Model file for the job. Use its own axes, mm. Face numbers are marked on the shaded views. Coordinates: 2 decimals unless noted, no trailing zeros. Write each loop counter-clockwise with the first axis right and the second up, starting at its lowest first coordinate (ties: lowest second). Pieces come first, ordered by that corner, then holes.
Q1. Pull direction Y, two halves, no side cores. Call the marked faces 1, 2, 3 and 4: released by +Y, released by -Y, zero draft, split by the parting line, or undercut.
Q2. Drill centre lines: probe 1 along Y at (x, z) = (755.5, 739); probe 2 along Y at (x, z) = (742, 731); probe 3 along X at (y, z) = (-300, 716.5). Where is each one in solid material? Low to high.
Q3. Band-saw the part on A-A, the plane y = -300. Write the cut outline in (x, z).
Q4. Band-saw the part on D-D, the plane x = 737. Write the cut outline in (y, z), plus the area to 3 significant figures.
Q5. Band-saw the part on C-C, the plane z = 742. Write the cut outline in (x, y).
Q6. Pin check, flat tips, straight feed: P1, Ø20, axis at y = -581, z = 729, coming from the -X side; P2, Ø4, axis at x = 744.5, z = 724, coming from the +Y side; P3, Ø6, axis at x = 750, y = -300, coming from the -Z side; P4, Ø12, axis at x = 744.5, y = -298, coming from the +Z side. Stop position of each tip, or through.
Q7. Band-saw the part on B-B, the plane z = 717. Write the cut outline in (x, y), plus the area to 3 significant figures.
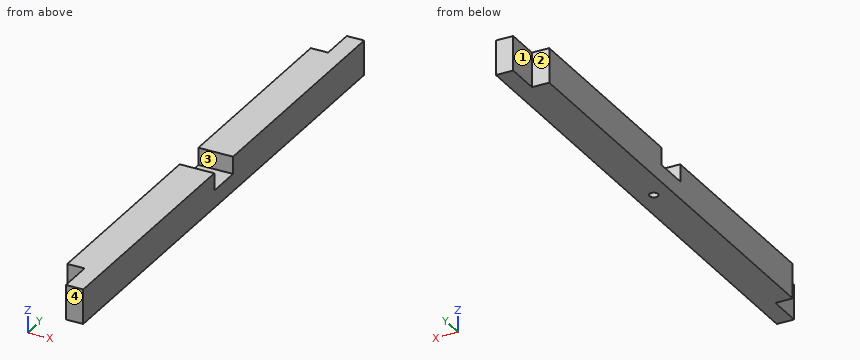
from build123d import *

# Parameters (mm, degrees)
SKETCH018_W     = 40
SKETCH018_H     = 40
PAD018_DEPTH    = 600
SKETCH019_W     = 40
SKETCH019_H     = 40
POCKET_DEPTH    = 20
SKETCH020_W     = 40
SKETCH020_H     = 40
POCKET001_DEPTH = 20
SKETCH064_R     = 5
POCKET019_DEPTH = 40.001


with BuildPart() as part:
    # Sketch018 → Pad018 (new body)
    with BuildSketch(Plane.XZ):
        with Locations((20, 280)):
            Rectangle(SKETCH018_W, SKETCH018_H)
    extrude(amount=PAD018_DEPTH)

    # Sketch019 (on Face4 of Pad018) → Pocket (cut)
    with BuildSketch(Plane(origin=(0, 0, 0), x_dir=(0, 0, -1), z_dir=(-1, 0, 0))):
        with Locations((-280, 580)):
            Rectangle(SKETCH019_W, SKETCH019_H)
        with Locations((-280, 20)):
            Rectangle(SKETCH019_W, SKETCH019_H)
    extrude(amount=-POCKET_DEPTH, mode=Mode.SUBTRACT)

    # Sketch020 (on Face1 of Pocket) → Pocket001 (cut)
    with BuildSketch(Plane(origin=(0, 0, 300), x_dir=(-1, 0, 0), z_dir=(0, 0, 1))):
        with Locations((-20, 300)):
            Rectangle(SKETCH020_W, SKETCH020_H)
    extrude(amount=-POCKET001_DEPTH, mode=Mode.SUBTRACT)

    # Sketch064 (on Face8 of Pocket001) → Pocket019 (cut, through all)
    with BuildSketch(Plane(origin=(0, 0, 260), x_dir=(1, 0, 0), z_dir=(0, 0, -1))):
        with Locations((20, 300)):
            Circle(SKETCH064_R)
    extrude(amount=-POCKET019_DEPTH, mode=Mode.SUBTRACT)


with BuildPart() as part_1:
    # Clone008 placement: moved
    add(part.part.moved(Location((730, 0, 0))))


with BuildPart() as part_2:
    # Clone012 placement: moved
    add(part_1.part.moved(Location((0, 0, 450))))


solid = part_2.part
Answer sheet:
1. face 1: zero draft
1. face 2: released by +Y
1. face 3: undercut
1. face 4: released by -Y
2. probe 1: y = -600 to -320, -280 to 0
2. probe 2: y = -560 to -320, -280 to -40
2. probe 3: x = 730 to 745, 755 to 770
3. outline: (730, 710) - (745, 710) - (745, 730) - (730, 730) - close; (755, 710) - (770, 710) - (770, 730) - (755, 730) - close
4. outline: (-560, 710) - (-40, 710) - (-40, 750) - (-280, 750) - (-280, 730) - (-320, 730) - (-320, 750) - (-560, 750) - close
4. area: 20,000 mm2
5. outline: (730, -560) - (750, -560) - (750, -600) - (770, -600) - (770, -320) - (730, -320) - close; (730, -280) - (770, -280) - (770, 0) - (750, 0) - (750, -40) - (730, -40) - close
6. P1: stops at x = 750
6. P2: stops at y = -40
6. P3: passes through
6. P4: stops at z = 730
7. outline: (730, -560) - (750, -560) - (750, -600) - (770, -600) - (770, 0) - (750, 0) - (750, -40) - (730, -40) - close; hole circle Ø10 at (750, -300)
7. area: 22,300 mm2
